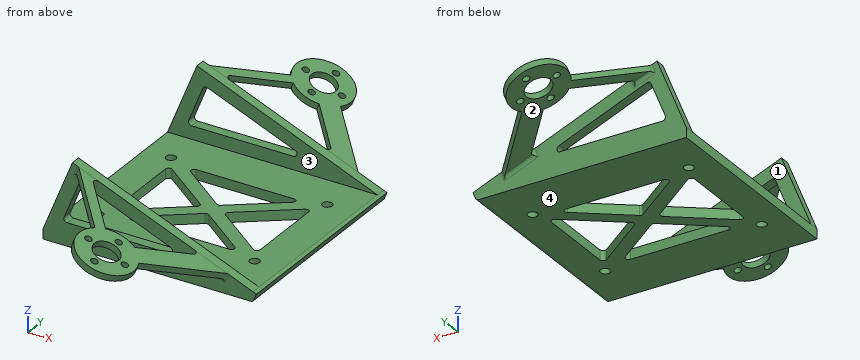
```python
from build123d import *

# Parameters (mm, degrees)
SKETCH_2_W          = 64.445610825
SKETCH_2_H          = 64.602792554
EXTRUDE_2_DEPTH     = 3
SKETCH_3_R          = 1.5
CUT_EXTRUDE_1_DEPTH = 4
EXTRUDE_3_DEPTH     = 3
EXTRUDE_4_DEPTH     = 3
EXTRUDE_6_DEPTH     = 64.602792554
SKETCH_11_R         = 1.05
SKETCH_11_R_2       = 4
EXTRUDE_7_DEPTH     = 2
FILLET_1_R          = 1
FILLET_2_R          = 1
FILLET_3_R          = 1
CUT_EXTRUDE_3_DEPTH = 75.557406075
FILLET_5_R          = 1


with BuildPart() as part:
    # 草图2 → 凸台-拉伸2 (new body)
    with BuildSketch(Plane.XY):
        with Locations((0.170214688, -0.018389364)):
            Rectangle(SKETCH_2_W, SKETCH_2_H)
    extrude(amount=EXTRUDE_2_DEPTH)

    # 草图3 → 切除-拉伸1 (cut)
    with BuildSketch(Plane.XY):
        with Locations((24, -18)):
            Circle(SKETCH_3_R)
        with Locations((-24, -18)):
            Circle(SKETCH_3_R)
        with Locations((-24, 18)):
            Circle(SKETCH_3_R)
        with Locations((24, 18)):
            Circle(SKETCH_3_R)
    extrude(amount=CUT_EXTRUDE_1_DEPTH, mode=Mode.SUBTRACT)

    # 草图9 → 凸台-拉伸3 (add)
    with BuildSketch(Plane(origin=(0, 32.283006913, 0), x_dir=(1, 0, 0), z_dir=(0, 1, 0))):
        Polygon((-32.052590724, -3), (32.393020101, -3), (-23.008931723, -25.383841499), align=None)
        Polygon((-20.798622679, -20.176679707), (11.814804037, -7), (-26.12234685, -7), align=None, mode=Mode.SUBTRACT)
    extrude(amount=-EXTRUDE_3_DEPTH)

    # 草图10 → 凸台-拉伸4 (add)
    with BuildSketch(Plane.XZ.offset(32.319785641)):
        Polygon((-23.008931723, 25.383841499), (-32.052590724, 3), (32.393020101, 3), align=None)
        Polygon((11.814804037, 7), (-20.798622679, 20.176679707), (-26.12234685, 7), align=None, mode=Mode.SUBTRACT)
    extrude(amount=-EXTRUDE_4_DEPTH)

    # 草图13 → 凸台-拉伸6 (add)
    with BuildSketch(Plane(origin=(0, 32.283006913, 0), x_dir=(1, 0, 0), z_dir=(0, 1, 0))):
        Polygon((32.393020101, -3), (33.435007656, -2.579009701), (32.393020101, 0), align=None)
    extrude(amount=-EXTRUDE_6_DEPTH)

    # 草图11 → 凸台-拉伸7 (add)
    # profile 1 of 2: a face of its own
    with BuildSketch(Plane(origin=(5.5877033, 0, 13.830050979), x_dir=(0.9271838545667869, 0, -0.37460659341591335), z_dir=(0.37460659341591335, 0, 0.9271838545667869))):
        with BuildLine():
            Line((-1.337035106, 45.610290293), (11.990248274, 32.283006913))
            Line((11.990248274, 32.283006913), (20.475529648, 32.283006913))
            Line((20.475529648, 32.283006913), (2.905605582, 49.85293098))
            ThreePointArc((2.905605582, 49.85293098), (-5.990504286, 62.698198683), (-12.551325133, 48.517320609))
            Line((-12.551325133, 48.517320609), (-28.785638829, 32.283006913))
            Line((-28.785638829, 32.283006913), (-24.542998142, 32.283006913))
            Line((-24.542998142, 32.283006913), (-10.430004789, 46.396000265))
            ThreePointArc((-10.430004789, 46.396000265), (-5.990504286, 44.76502259), (-1.337035106, 45.610290293))
        make_face()
        with Locations((0.784285238, 53.731610636)):
            Circle(SKETCH_11_R, mode=Mode.SUBTRACT)
        with Locations((-11.215714762, 53.731610636)):
            Circle(SKETCH_11_R, mode=Mode.SUBTRACT)
        with Locations((-5.215714762, 47.731610636)):
            Circle(SKETCH_11_R, mode=Mode.SUBTRACT)
        with Locations((-5.215714762, 53.731610636)):
            Circle(SKETCH_11_R_2, mode=Mode.SUBTRACT)
        with Locations((-5.215714762, 59.731610636)):
            Circle(SKETCH_11_R, mode=Mode.SUBTRACT)
    # profile 2 of 2: a face of its own
    with BuildSketch(Plane(origin=(5.5877033, 0, 13.830050979), x_dir=(0.9271838545667869, 0, -0.37460659341591335), z_dir=(0.37460659341591335, 0, 0.9271838545667869))):
        with BuildLine():
            Line((11.990248274, -32.319785641), (-1.337035106, -45.64706902))
            ThreePointArc((-1.337035106, -45.64706902), (-5.990504286, -44.801801317), (-10.430004789, -46.432778993))
            Line((-10.430004789, -46.432778993), (-24.542998142, -32.319785641))
            Line((-24.542998142, -32.319785641), (-28.785638829, -32.319785641))
            Line((-28.785638829, -32.319785641), (-12.551325133, -48.554099337))
            ThreePointArc((-12.551325133, -48.554099337), (-5.990504286, -62.73497741), (2.905605582, -49.889709707))
            Line((2.905605582, -49.889709707), (20.475529648, -32.319785641))
            Line((20.475529648, -32.319785641), (11.990248274, -32.319785641))
        make_face()
        with Locations((0.784285238, -53.768389364)):
            Circle(SKETCH_11_R, mode=Mode.SUBTRACT)
        with Locations((-11.215714762, -53.768389364)):
            Circle(SKETCH_11_R, mode=Mode.SUBTRACT)
        with Locations((-5.215714762, -59.768389364)):
            Circle(SKETCH_11_R, mode=Mode.SUBTRACT)
        with Locations((-5.215714762, -53.768389364)):
            Circle(SKETCH_11_R_2, mode=Mode.SUBTRACT)
        with Locations((-5.215714762, -47.768389364)):
            Circle(SKETCH_11_R, mode=Mode.SUBTRACT)
    extrude(amount=-EXTRUDE_7_DEPTH)

    # 圆角1
    fillet_1_edges = [part.edges().sort_by_distance(p)[0] for p in [
        (32.393020101, -0.018389364, 0),
    ]]
    fillet(fillet_1_edges, radius=FILLET_1_R)

    # 圆角2
    fillet_2_edges = [part.edges().sort_by_distance(p)[0] for p in [
        (16.330261319, -32.319785641, 8.411241064),
        (24.19767721, -32.319785641, 5.232598715),
        (-21.476482859, -32.319785641, 23.686157226),
        (-17.542774913, -32.319785641, 22.096836051),
        (19.889362671, -32.319785641, 5.894736035),
        (-19.884235479, -32.319785641, 21.964312784),
        (24.19767721, 32.283006913, 5.232598715),
        (16.330261319, 32.283006913, 8.411241064),
        (-17.542774913, 32.283006913, 22.096836051),
        (-21.476482859, 32.283006913, 23.686157226),
        (19.889362671, 32.283006913, 5.894736035),
        (-19.884235479, 32.283006913, 21.964312784),
    ]]
    fillet(fillet_2_edges, radius=FILLET_2_R)

    # 圆角3
    fillet_3_edges = [part.edges().sort_by_distance(p)[0] for p in [
        (-26.12234685, 30.783006913, 7),
        (11.814804037, 30.783006913, 7),
        (-20.798622679, 30.783006913, 20.176679707),
        (-26.12234685, -30.819785641, 7),
        (-20.798622679, -30.819785641, 20.176679707),
        (11.814804037, -30.819785641, 7),
    ]]
    fillet(fillet_3_edges, radius=FILLET_3_R)

    # 草图15 → 切除-拉伸3 (cut, through all)
    with BuildSketch(Plane.XY.offset(3)):
        Polygon((-18, 16), (18, 16), (0, 2.5), align=None)
        Polygon((-22, 14), (-3.333333333, 0), (-22, -14), align=None)
        Polygon((-18, -16), (18, -16), (0, -2.5), align=None)
        Polygon((22, 14), (3.333333333, 0), (22, -14), align=None)
    extrude(amount=-CUT_EXTRUDE_3_DEPTH, mode=Mode.SUBTRACT)

    # 圆角5
    fillet_5_edges = [part.edges().sort_by_distance(p)[0] for p in [
        (-18, -16, 1.5),
        (0, -2.5, 1.5),
        (18, -16, 1.5),
        (-22, -14, 1.5),
        (-22, 14, 1.5),
        (-3.333333333, 0, 1.5),
        (22, 14, 1.5),
        (22, -14, 1.5),
        (3.333333333, 0, 1.5),
        (0, 2.5, 1.5),
        (-18, 16, 1.5),
        (18, 16, 1.5),
    ]]
    fillet(fillet_5_edges, radius=FILLET_5_R)


solid = part.part
```
Geometry: final body of the model. Coordinates: model frame, mm. Face numbers are marked on the shaded views. A direction names the side the tool comes from. Coordinates: 2 decimals unless noted, no trailing zeros. Loops run counter-clockwise (first coordinate to the right, second up) from the corner with the lowest first, then second, coordinate; pieces in that order, holes last. Notation, with made-up numbers: M -35.75,51.25 L -30.75,51.25 A16 ccw -30.75,62.25 Z; hole C -31,43 d5. An arc over 180 degrees is marked long. Put each result on its own line as item: value.
(1) Cut plane A-A on y = 18. Return the cut outline in (x, z) (3 decimals), then the cut area to 3 significant figures.
Answer sheet:
outline: M -32.053,0 L -25.5,0 L -25.5,3 L -32.053,3 Z; M -22.5,0 L 22.5,0 L 22.5,3 L -22.5,3 Z; M 25.5,0 L 31.719,0 A1 ccw 32.646,0.625 L 33.435,2.579 L 32.393,3 L 25.5,3 Z
area: 177 mm^2
(2) Cut plane B-B on x = -13.5. State how many separate pieces and enclosed holes the cut face has, then the cut area to 3 significant figures.
Answer sheet:
separate pieces: 8
enclosed holes: 0
area: 196 mm^2
(3) Material intervals for probe 1 along Y at (x, z) = (-24, 1.7); probe 2 along Y at (x, z) = (-9.5, 3.25); probe 3 along X at (y, z) = (-18, 1.5), sorted ascending.
Answer sheet:
probe 1: y = -32.32 to -19.5, -16.5 to 16.5, 19.5 to 32.28
probe 2: y = -32.32 to -29.32, 29.28 to 32.28
probe 3: x = -32.05 to -25.5, -22.5 to 22.5, 25.5 to 33
(4) Access query for the marked faces 1 and 2. Directions: +Z, -Z, +X, -X, +Y, -Y. A direction counts if a zero-diameter tool reaches every point of the face in a straight line with its end or side. Return the directions, or none.
Answer sheet:
face 1: +Z, +X, -X
face 2: -Z, -X, +Y
(5) Draft query along Y for the marked faces 3 and 4. Return one class per face: pulls with the +Y half, pulls with the -Y half, needs draft (parallel to the pull), parting line crosses it, or undercut.
Answer sheet:
face 3: undercut
face 4: needs draft
(6) First-contact query: pin 1 (1.5 mm diameter, centred on x = -1.5, z = 1, fed in from -Y); pin 2 (3.5 mm diameter, centred on x = -24, y = 18, fed in from +Z); pin 3 (3.5 mm diameter, centred on x = -10, y = 30, fed in from +Z). Flat tips, straight axial feed; report the tip coordinate or a pass-through.
Answer sheet:
pin 1: stops at y = -32.32
pin 2: stops at z = 3
pin 3: stops at z = 20.83
